```python
from build123d import *

# Parameters (mm, degrees)
BOSS_EXTRUDE1_DEPTH = 10
SKETCH4_R           = 1.75
CUT_EXTRUDE2_DEPTH  = 21.287003229


with BuildPart() as part:
    # Sketch1 → Boss-Extrude1 (new body)
    with BuildSketch(Plane(origin=(0, 0, 0), x_dir=(1, 0, 0), z_dir=(0, 1, 0))):
        with BuildLine():
            Line((17, 4), (-5, 4))
            Line((-5, 4), (-5, -0.75))
            Line((-5, -0.75), (1.104356076, -0.75))
            Line((1.104356076, -0.75), (1.104356076, 0))
            ThreePointArc((1.104356076, 0), (2.25, 1.75), (3.395643924, 0))
            Line((3.395643924, 0), (3.395643924, -0.75))
            Line((3.395643924, -0.75), (5.104356076, -0.75))
            Line((5.104356076, -0.75), (5.104356076, 0))
            ThreePointArc((5.104356076, 0), (6.25, 1.75), (7.395643924, 0))
            Line((7.395643924, 0), (7.395643924, -0.75))
            Line((7.395643924, -0.75), (9.104356076, -0.75))
            Line((9.104356076, -0.75), (9.104356076, 0))
            ThreePointArc((9.104356076, 0), (10.25, 1.75), (11.395643924, 0))
            Line((11.395643924, 0), (11.395643924, -0.75))
            Line((11.395643924, -0.75), (13.104356076, -0.75))
            Line((13.104356076, -0.75), (13.104356076, 0))
            ThreePointArc((13.104356076, 0), (14.25, 1.75), (15.395643924, 0))
            Line((15.395643924, 0), (15.395643924, -0.75))
            Line((15.395643924, -0.75), (17, -0.75))
            Line((17, -0.75), (17, 4))
        make_face()
    extrude(amount=BOSS_EXTRUDE1_DEPTH)

    # Sketch4 → Cut-Extrude2 (cut, through all)
    with BuildSketch(Plane.XY.offset(0.75)):
        with Locations((-1.947821962, 5)):
            Circle(SKETCH4_R)
    extrude(amount=-CUT_EXTRUDE2_DEPTH, mode=Mode.SUBTRACT)


solid = part.part
```
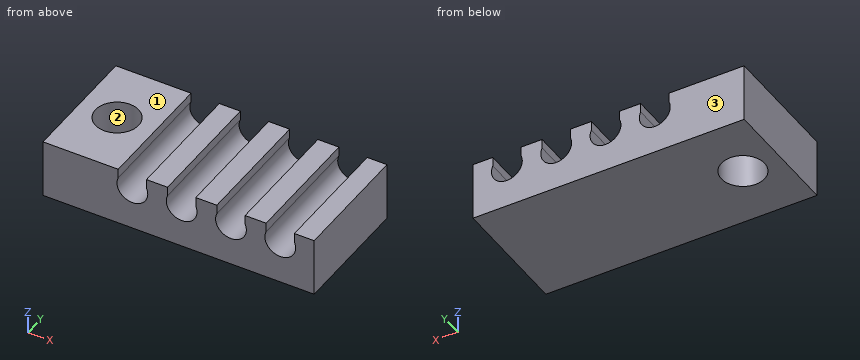
The model under review builds one solid part; all positions refer to its coordinate system, in mm. Face numbers are marked on the shaded views. Give positions to 0.01 mm unless a question says otherwise; leave off trailing zeros. Write each loop counter-clockwise with the first axis right and the second up, starting at its lowest first coordinate (ties: lowest second). Pieces come first, ordered by that corner, then holes. Notation, with made-up numbers: M 27,40.5 L 41,40.5 A35 ccw 41,75.5 Z; hole C -22.5,-11 d8. An arc over 180 degrees is marked long. Answer in a Markdown table with one row per item.
Item 1: Add section D-D on z = -2.85. Give the boundary of the cut face in (x, y), plus the area to 3 significant figures.
Check sheet entries:
| item | result |
|---|---|
| outline | M -5,0 L 17,0 L 17,10 L -5,10 Z; hole C -1.95,5 d3.5 |
| area | 210 mm2 |
Item 2: Add section A-A on y = 5. Give the boundary of the cut face in (x, z), plus the area to 3 significant figures.
Check sheet entries:
| item | result |
|---|---|
| outline | M -5,-4 L -3.7,-4 L -3.7,0.75 L -5,0.75 Z; M -0.2,-4 L 17,-4 L 17,0.75 L 15.4,0.75 L 15.4,0 A1.25 cw long 13.1,0 L 13.1,0.75 L 11.4,0.75 L 11.4,0 A1.25 cw long 9.1,0 L 9.1,0.75 L 7.4,0.75 L 7.4,0 A1.25 cw long 5.1,0 L 5.1,0.75 L 3.4,0.75 L 3.4,0 A1.25 cw long 1.1,0 L 1.1,0.75 L -0.2,0.75 Z |
| area | 66.3 mm2 |
Item 3: Draft analysis for pull direction Y (two halves, no side actions). For the marked faces 1, 2 and 3, state which applies: +Y half, -Y half, draft (parallel to the pull), parting line (faces both ways), or undercut.
Check sheet entries:
| item | result |
|---|---|
| face 1 | draft |
| face 2 | undercut |
| face 3 | +Y half |
Item 4: For line 1 along X through (y, z) = (7.5, -0.5); line 2 along X through (y, z) = (4.25, -0.25); line 3 along X through (y, z) = (1.75, -1.5), list the stretches that pass through material, from the lowest coordinate up.
Check sheet entries:
| item | result |
|---|---|
| line 1 | -5 to 1, 3.5 to 5, 7.5 to 9, 11.5 to 13, 15.5 to 17 |
| line 2 | -5 to -3.53, -0.37 to 1.03, 3.47 to 5.03, 7.47 to 9.03, 11.47 to 13.03, 15.47 to 17 |
| line 3 | -5 to 1.5, 3 to 5.5, 7 to 9.5, 11 to 13.5, 15 to 17 |
Item 5: Add section B-B on z = -1.45. Give the boundary of the cut face in (x, y).
Check sheet entries:
| item | result |
|---|---|
| outline | M -5,0 L 1.44,0 L 1.44,10 L -5,10 Z; M 3.06,0 L 5.44,0 L 5.44,10 L 3.06,10 Z; M 7.06,0 L 9.44,0 L 9.44,10 L 7.06,10 Z; M 11.06,0 L 13.44,0 L 13.44,10 L 11.06,10 Z; M 15.06,0 L 17,0 L 17,10 L 15.06,10 Z; hole C -1.95,5 d3.5 |
Item 6: Add section C-C on x = -0.5. Give the boundary of the cut face in (y, z).
Check sheet entries:
| item | result |
|---|---|
| outline | M 0,-4 L 4.02,-4 L 4.02,0.75 L 0,0.75 Z; M 5.98,-4 L 10,-4 L 10,0.75 L 5.98,0.75 Z |
